```python
from build123d import *

# Parameters (mm, degrees)
SKETCH1_W           = 20
SKETCH1_H           = 5
BOSS_EXTRUDE1_DEPTH = 1.5
SKETCH2_W           = 2.9
SKETCH2_H           = 2.9
SKETCH2_W_2         = 2.8
SKETCH2_H_2         = 2.8
SKETCH2_W_3         = 2.7
SKETCH2_H_3         = 2.7
SKETCH2_W_4         = 2.6
SKETCH2_H_4         = 2.6
BOSS_EXTRUDE2_DEPTH = 5


with BuildPart() as part:
    # Sketch1 → Boss-Extrude1 (new body)
    with BuildSketch(Plane.XY):
        with Locations((10, 2.5)):
            Rectangle(SKETCH1_W, SKETCH1_H)
    extrude(amount=BOSS_EXTRUDE1_DEPTH)

    # Sketch2 → Boss-Extrude2 (add)
    with BuildSketch(Plane.XY.offset(1.5)):
        with Locations((2.5, 2.5)):
            Rectangle(SKETCH2_W, SKETCH2_H)
        with Locations((7.35, 2.5)):
            Rectangle(SKETCH2_W_2, SKETCH2_H_2)
        with Locations((12.1, 2.5)):
            Rectangle(SKETCH2_W_3, SKETCH2_H_3)
        with Locations((16.75, 2.5)):
            Rectangle(SKETCH2_W_4, SKETCH2_H_4)
    extrude(amount=BOSS_EXTRUDE2_DEPTH)


solid = part.part
```
Work out the finished part from the listing and answer in its coordinate system (mm). A direction names the side the tool comes from. Coordinates: 2 decimals unless noted, no trailing zeros. Write each loop counter-clockwise with the first axis right and the second up, starting at its lowest first coordinate (ties: lowest second). Pieces come first, ordered by that corner, then holes.
Q1. A cutting plane is placed at D-D, the plane x = 6.5. Give the vertices of the cut face in (y, z).
Q2. A cutting plane is placed at A-A, the plane z = 2.25. Give the vertices of the cut face in (x, y).
Q3. Each of these flat-tipped pins is pushed along its axis until it touches: pin 1 Ø2.5 at (x, z) = (2.5, 3) entering from +Y; pin 2 Ø3 at (y, z) = (2.5, 4) entering from -X; pin 3 Ø1.4 at (y, z) = (2, 4) entering from +X. Where does it stop, or does it pass through?
Q4. Find the intervals of material crossed by line 1 (X direction, y = 3.7, z = 4.5); line 2 (Y direction, x = 8.5, z = 2.5); line 3 (Y direction, x = 1.5, z = 5.75), in increasing order.
Q5. A cutting plane is placed at C-C, the plane y = 3.2. Give the vertices of the cut face in (x, z), then the cut area to 3 significant figures.
Q6. Which of the six approach directions +Z, -Z, +X, -X, +Y, -Y give full straight-line access (tool end or side, diameter ignored) to faces 1 (the face through (17, 1.2, 4)), 2 (the face through (2, 1.05, 4)), 3 (the face through (3.95, 2, 4)), 4 (the face through (12, 3.85, 4))?
Q7. A cutting plane is placed at B-B, the plane x = 1.75. Give the vertices of the cut face in (y, z), then the cut area to 3 significant figures.
Findings below:
1. outline: (0, 0) - (5, 0) - (5, 1.5) - (3.9, 1.5) - (3.9, 6.5) - (1.1, 6.5) - (1.1, 1.5) - (0, 1.5) - close
2. outline: (1.05, 1.05) - (3.95, 1.05) - (3.95, 3.95) - (1.05, 3.95) - close; (5.95, 1.1) - (8.75, 1.1) - (8.75, 3.9) - (5.95, 3.9) - close; (10.75, 1.15) - (13.45, 1.15) - (13.45, 3.85) - (10.75, 3.85) - close; (15.45, 1.2) - (18.05, 1.2) - (18.05, 3.8) - (15.45, 3.8) - close
3. pin 1: stops at y = 3.95
3. pin 2: stops at x = 1.05
3. pin 3: stops at x = 18.05
4. line 1: x = 1.05 to 3.95, 5.95 to 8.75, 10.75 to 13.45, 15.45 to 18.05
4. line 2: y = 1.1 to 3.9
4. line 3: y = 1.05 to 3.95
5. outline: (0, 0) - (20, 0) - (20, 1.5) - (18.05, 1.5) - (18.05, 6.5) - (15.45, 6.5) - (15.45, 1.5) - (13.45, 1.5) - (13.45, 6.5) - (10.75, 6.5) - (10.75, 1.5) - (8.75, 1.5) - (8.75, 6.5) - (5.95, 6.5) - (5.95, 1.5) - (3.95, 1.5) - (3.95, 6.5) - (1.05, 6.5) - (1.05, 1.5) - (0, 1.5) - close
5. area: 85.0 mm2
6. face 1: +Z, +X, -Y
6. face 2: +Z, +X, -X, -Y
6. face 3: +Z, +Y, -Y
6. face 4: +Z, +X, +Y
7. outline: (0, 0) - (5, 0) - (5, 1.5) - (3.95, 1.5) - (3.95, 6.5) - (1.05, 6.5) - (1.05, 1.5) - (0, 1.5) - close
7. area: 22.0 mm2
